Autodesk Inventor part; units mm, degrees
ref_plane "YZ Plane" through (0, 0, 0) normal (1, 0, 0) x (0, 1, 0)
ref_plane "XZ Plane" through (0, 0, 0) normal (0, 1, 0) x (-1, 0, 0)
ref_plane "XY Plane" through (0, 0, 0) normal (0, 0, 1) x (1, 0, 0)
sketch "Sketch1" plane through (0, 0, 0) normal (0, 0, 1) x (1, 0, 0)
  line L0 (0, 66.5) -> (0, -66.5) construction
  line L1 (-42, 0) -> (42, 0) construction
  line L2 (30, -47.5) -> (-30, -47.5)
  line L3 (-30, -47.5) -> (-30, 47.5)
  line L4 (-30, 47.5) -> (30, 47.5)
  line L5 (30, 47.5) -> (30, -47.5)
  line L6 (30, -47.5) -> (-30, 47.5) construction
  line L7 (-30, -47.5) -> (30, 47.5) construction
  line L8 (5.5, 2) -> (-15.5, 2)
  line L9 (-15.5, 2) -> (-15.5, 33)
  line L10 (-15.5, 33) -> (5.5, 33)
  line L11 (5.5, 33) -> (5.5, 2)
  line L12 (5.5, 2) -> (-15.5, 33) construction
  line L13 (-15.5, 2) -> (5.5, 33) construction
  line L14 (15.5, -33) -> (-5.5, -33)
  line L15 (-5.5, -33) -> (-5.5, -2)
  line L16 (-5.5, -2) -> (15.5, -2)
  line L17 (15.5, -2) -> (15.5, -33)
  line L18 (15.5, -33) -> (-5.5, -2) construction
  line L19 (-5.5, -33) -> (15.5, -2) construction
  point P0 (0, 0)
  point P1 (-5, 17.5)
  point P2 (5, -17.5)
  dimension "d13" = 95
  dimension "d14" = 60
  dimension "d15" = 31
  dimension "d16" = 21
  dimension "d17" = 5
  dimension "d18" = 17.5
  dimension "d19" = 17.5
  dimension "d20" = 5
extrude "Extrusion3" add sketch "Sketch1" along normal blind 2
sketch "Sketch2" plane through (0, 0, 2) normal (0, 0, 1) x (1, 0, 0)
  line L0 (25, -37.5) -> (-25, -37.5) construction
  line L1 (-25, -37.5) -> (-25, 37.5) construction
  line L2 (-25, 37.5) -> (25, 37.5) construction
  line L3 (25, 37.5) -> (25, -37.5) construction
  line L4 (25, -37.5) -> (-25, 37.5) construction
  line L5 (-25, -37.5) -> (25, 37.5) construction
  point P0 (0, 0)
  point P1 (-25, -37.5)
  dimension "d21" = 75
  dimension "d22" = 50
hole "Hole1" at (25, 37.5, 2) at (-25, -37.5, 2) direction (0, 0, -1) diameter 3.2 end through all
fillet "Fillet1" radius 5 4 edges at (30, 47.5, 1) (-30, 47.5, 1) (30, -47.5, 1) (-30, -47.5, 1)
properties part number "17-0028-0112" material "Plastic (perspex PMMA)"
Here's how the part is built. I have some questions about the finished solid (model axes, mm). A direction names the side the tool comes from. Coordinates: 2 decimals unless noted, no trailing zeros. Order: outer loops, then holes, each group sorted by start corner. A loop starts at its lowest first (then second) coordinate and runs counter-clockwise, first axis right, second up. Notation, with made-up numbers: (-19, 18) -> (38, 18) arc R17 ccw to (38, 51) -> close; hole circle Ø2 at (-38.5, -22). An arc over 180 degrees is marked (long way). Return JSON: item names as keys, results as strings.
1) If we section it at D-D on y = -37.5: List the corners of the cut face in (x, z) for me, plus the area to 3 significant figures.
Conclusion:
{"outline": "(-30, 0) -> (-26.6, 0) -> (-26.6, 2) -> (-30, 2) -> close; (-23.4, 0) -> (30, 0) -> (30, 2) -> (-23.4, 2) -> close", "area": "114 mm²"}
2) If we section it at A-A on x = 1: List the corners of the cut face in (y, z) for me.
Conclusion:
{"outline": "(-47.5, 0) -> (-33, 0) -> (-33, 2) -> (-47.5, 2) -> close; (-2, 0) -> (2, 0) -> (2, 2) -> (-2, 2) -> close; (33, 0) -> (47.5, 0) -> (47.5, 2) -> (33, 2) -> close"}
3) If we section it at C-C on z = 1.7: List the corners of the cut face in (x, y) for me, plus the area to 3 significant figures.
Conclusion:
{"outline": "(-30, -42.5) arc R5 ccw to (-25, -47.5) -> (25, -47.5) arc R5 ccw to (30, -42.5) -> (30, 42.5) arc R5 ccw to (25, 47.5) -> (-25, 47.5) arc R5 ccw to (-30, 42.5) -> close; hole circle Ø3.2 at (-25, -37.5); hole (-15.5, 2) -> (5.5, 2) -> (5.5, 33) -> (-15.5, 33) -> close; hole (-5.5, -33) -> (15.5, -33) -> (15.5, -2) -> (-5.5, -2) -> close; hole circle Ø3.2 at (25, 37.5)", "area": "4,360 mm²"}
4) If we section it at B-B on y = 29: List the corners of the cut face in (x, z) for me.
Conclusion:
{"outline": "(-30, 0) -> (-15.5, 0) -> (-15.5, 2) -> (-30, 2) -> close; (5.5, 0) -> (30, 0) -> (30, 2) -> (5.5, 2) -> close"}
5) On a 3-axis mill with a long thin cutter (end or side, diameter ignored), from which of +Z, -Z, +X, -X, +Y, -Y can I reach the whole of each face in a straight line? I mean faces 1 (the flat face through (15.5, -17, 1)), 2 (the flat face through (30, 1, 1)). Say none if no direction works.
Conclusion:
{"face 1": "+Z, -Z", "face 2": "+Z, -Z, +X, +Y, -Y"}
6) If I drill on probe 1 along Y at (x, z) = (-2, 0.4); probe 2 along X at (y, z) = (-11, 0.8); probe 3 along X at (y, z) = (37.5, 0.5), over which ranges is the centre line in solid material (lowest first)?
Conclusion:
{"probe 1": "y = -47.5 to -33, -2 to 2, 33 to 47.5", "probe 2": "x = -30 to -5.5, 15.5 to 30", "probe 3": "x = -30 to 23.4, 26.6 to 30"}
